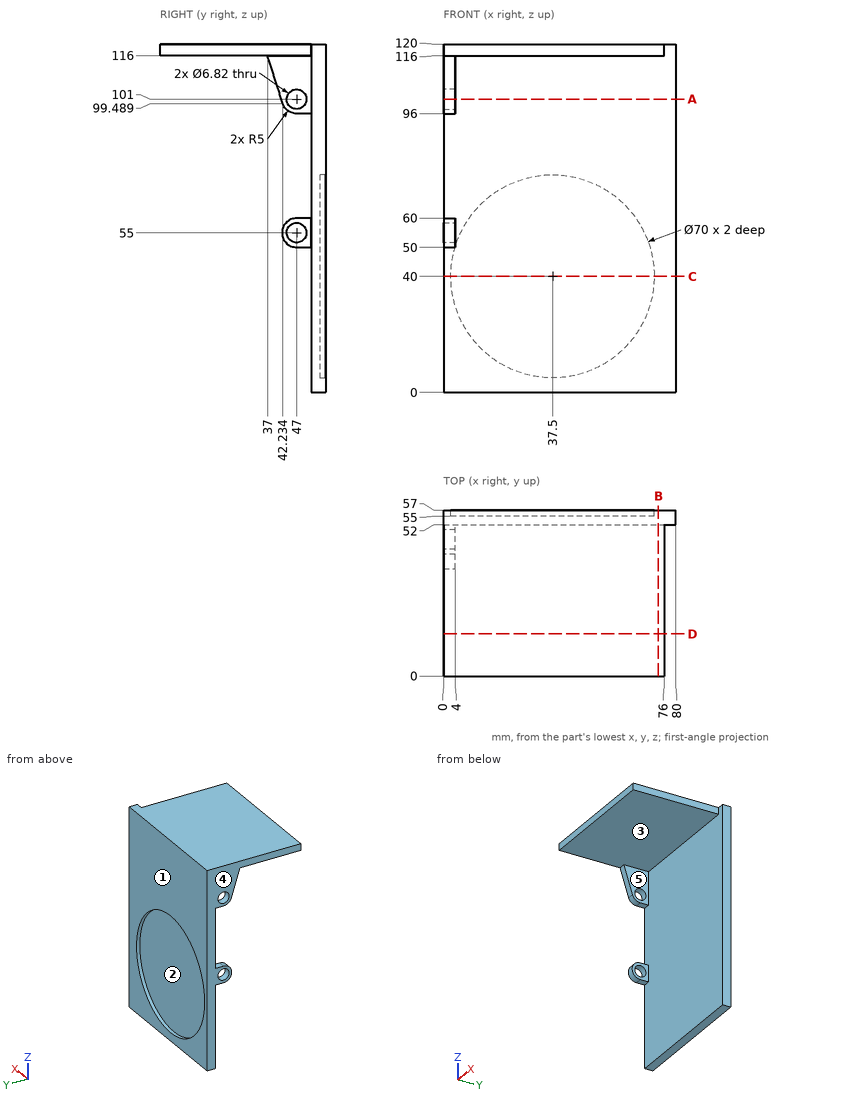
Design review of the part shown in the three views and the two pictorial views. Dimensions are in mm from the part's minimum x, y and z. A direction names the side the tool comes from. Give positions to 0.01 mm unless a question says otherwise; leave off trailing zeros. Loops run counter-clockwise (first coordinate to the right, second up) from the corner with the lowest first, then second, coordinate; pieces in that order, holes last. Notation, with made-up numbers: (-37.5, 44.25) -> (-22.5, 44.25) arc R14 ccw to (-22.5, 55.25) -> close; hole circle Ø2 at (61, -5.75). An arc over 180 degrees is marked (long way). Answer as a JSON object with one key per item and string values. Group by question number.
Q1. Take a section at C-C (z = 40). Write out the cut boundary in (x, y).
Q2. Tool access review of the marked faces 4 and 5: name each direction out of +Z, -Z, +X, -X, +Y, -Y from which nothing blocks a thin tool from reaching the whole face with its end or side.
Q3. Take a section at D-D (y = 14.5). Write out the cut boundary in (x, z), plus the area to 3 significant figures.
Q4. Take a section at A-A (z = 101). Write out the cut boundary in (x, y) (1 decimal), plus the area to 3 significant figures.
Q5. Insertion check: pin 1 (2 mm diameter, centred on x = 2.5, y = 48.5, fed in from -Z); pin 2 (15.5 mm diameter, centred on x = 40, y = 20.5, fed in from -Z); pin 3 (4.5 mm diameter, centred on y = 47.5, z = 109.5, fed in from +X). Each pin has a flat end and moves straight along its axis. Give the tip position at first contact, or say it passes through.
Q6. Take a section at B-B (x = 74). Write out the cut boundary in (y, z), plus the area to 3 significant figures.
Q7. Draft analysis for pull direction Z (two halves, no side actions). For the marked faces 1, 2 and 3, state which applies: pulls with the +Z half, pulls with the -Z half, needs draft (parallel to the pull), parting line crosses it, or undercut.
Q8. Wall thickness on line 1 along Z through (x, y) = (37, 56); line 2 along Y through (x, z) = (2.05, 55); line 3 along Y through (x, z) = (43, 30): over which ranges is each line inside the solid? List them lowest first.
Answer below:
{
 "1": {"outline": "(0, 52) -> (80, 52) -> (80, 57) -> (72.5, 57) -> (72.5, 55) -> (2.5, 55) -> (2.5, 57) -> (0, 57) -> close"},
 "2": {"face 4": "+Z, -Z, -X, +Y, -Y", "face 5": "-Z, +X, -Y"},
 "3": {"outline": "(0, 116) -> (76, 116) -> (76, 120) -> (0, 120) -> close", "area": "304 mm2"},
 "4": {"outline": "(0, 41.8) -> (4, 41.8) -> (4, 43.6) -> (0, 43.6) -> close; (0, 50.4) -> (4, 50.4) -> (4, 52) -> (80, 52) -> (80, 57) -> (0, 57) -> close", "area": "414 mm2"},
 "5": {"pin 1": "stops at z = 50", "pin 2": "stops at z = 116", "pin 3": "stops at x = 4"},
 "6": {"outline": "(0, 116) -> (52, 116) -> (52, 0) -> (57, 0) -> (57, 120) -> (0, 120) -> close", "area": "808 mm2"},
 "7": {"face 1": "needs draft", "face 2": "undercut", "face 3": "pulls with the -Z half"},
 "8": {"line 1": "z = 0 to 5, 75 to 120", "line 2": "y = 42 to 43.59, 50.41 to 57", "line 3": "y = 52 to 55"}
}
